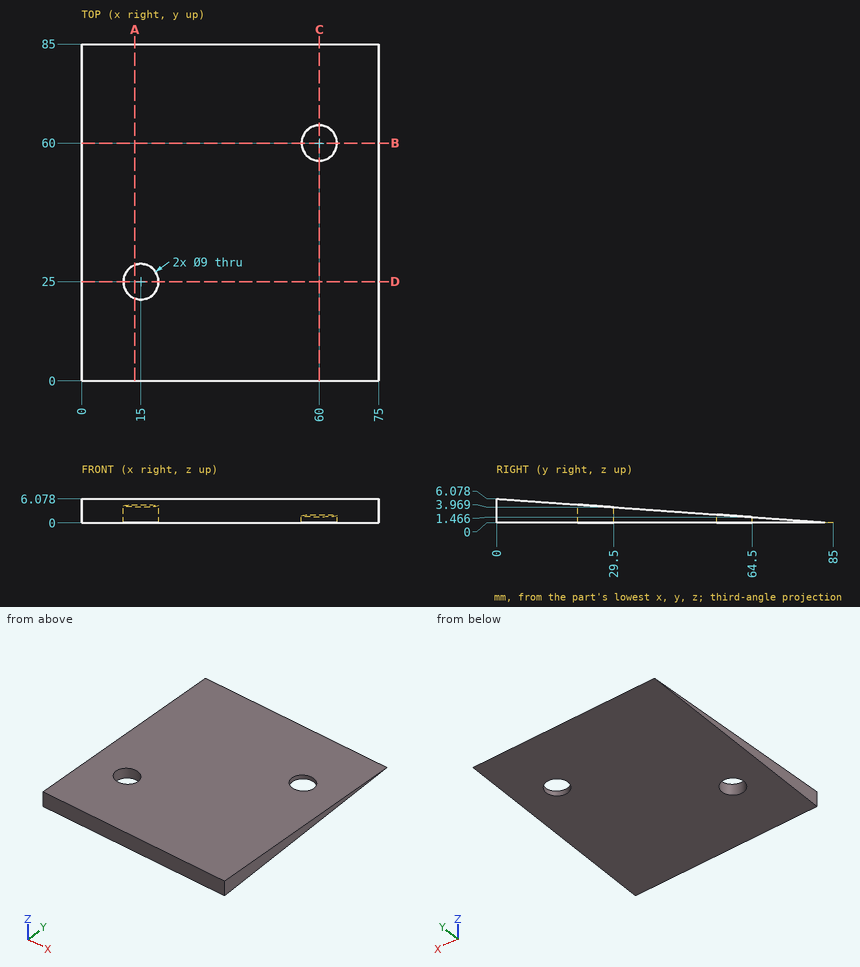
Geometry: see drawing. Coordinates: mm, zero at the bounding-box minimum. Round coordinates to 2 decimals unless told otherwise and drop trailing zeros. Write each loop counter-clockwise with the first axis right and the second up, starting at its lowest first coordinate (ties: lowest second). Pieces come first, ordered by that corner, then holes. Notation, with made-up numbers: (-13, 24.5) -> (21, 24.5) arc R13 cw to (21, 30.5) -> close; hole circle Ø1 at (79, 15.25). An arc over 180 degrees is marked (long way). Answer as CSV lines item,"result".
1. Section D-D (y = 25). Return the cut outline in (x, z), plus the area to 3 significant figures.
Geometry says:
outline,"(0, 0) -> (10.5, 0) -> (10.5, 4.29) -> (0, 4.29) -> close; (19.5, 0) -> (75, 0) -> (75, 4.29) -> (19.5, 4.29) -> close"
area,"283 mm^2"
2. Section A-A (x = 13.5). Return the cut outline in (y, z), plus the area to 3 significant figures.
Geometry says:
outline,"(0, 0) -> (20.76, 0) -> (20.76, 4.59) -> (0, 6.08) -> close; (29.24, 0) -> (85, 0) -> (29.24, 3.99) -> close"
area,"222 mm^2"
3. Section B-B (y = 60). Return the cut outline in (x, z).
Geometry says:
outline,"(0, 0) -> (55.5, 0) -> (55.5, 1.79) -> (0, 1.79) -> close; (64.5, 0) -> (75, 0) -> (75, 1.79) -> (64.5, 1.79) -> close"
4. Contact query for flat-ended pins moving along their axis: P1, Ø12, axis at x = 63, y = 53.5, coming from the +Z side; P2, Ø14.5, axis at x = 60, y = 60, coming from the +Z side; P3, Ø7, axis at x = 15, y = 25, coming from the -Z side. Output: stop coordinate, or through.
Geometry says:
P1,"stops at z = 2.68"
P2,"stops at z = 2.31"
P3,"passes through"
5. Ray query, L1, parallel to X at y = 25, z = 3.3; L2, parallel to X at y = 60, z = 0.9; L3, parallel to Z at x = 63, y = 25. Return the intervals inside material, ascending. Write a range as [from, to].
Geometry says:
L1,"x = [0, 10.5], [19.5, 75]"
L2,"x = [0, 55.5], [64.5, 75]"
L3,"z = [0, 4.29]"
6. Section C-C (x = 60). Return the cut outline in (y, z), plus the area to 3 significant figures.
Geometry says:
outline,"(0, 0) -> (55.5, 0) -> (55.5, 2.11) -> (0, 6.08) -> close; (64.5, 0) -> (85, 0) -> (64.5, 1.47) -> close"
area,"242 mm^2"
